Work out the finished part from the listing and answer in its coordinate system (mm). Face numbers are marked on the shaded views. A direction names the side the tool comes from. Round coordinates to 2 decimals unless told otherwise and drop trailing zeros. Loops run counter-clockwise (first coordinate to the right, second up) from the corner with the lowest first, then second, coordinate; pieces in that order, holes last. Notation, with made-up numbers: (23.25, -23.5) -> (38.25, -23.5) arc R24 cw to (38.25, 11.5) -> close; hole circle Ø8 at (59.5, -20.75). An arc over 180 degrees is marked (long way). Use one line per item in the form item = value.
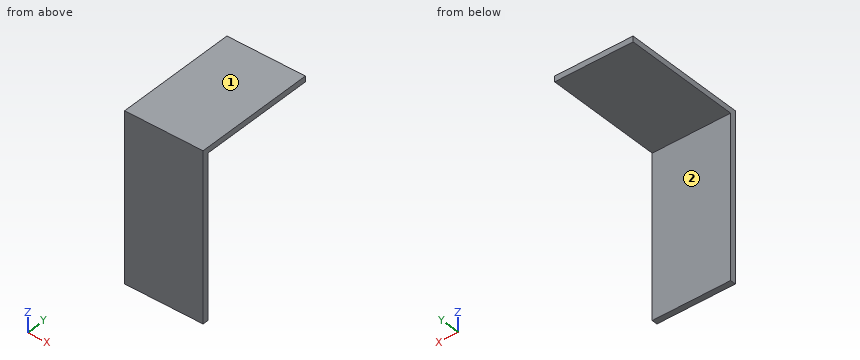
```python
from build123d import *

# Parameters (mm, degrees)
F0_W     = 250
F0_H     = 517
F1_DEPTH = 18
F2_W     = 250
F2_H     = 18
F3_DEPTH = 390


with BuildPart() as f1:
    # F0 (on Front) → F1 (new body)
    with BuildSketch(Plane.XZ):
        with Locations((125, 258.5)):
            Rectangle(F0_W, F0_H)
    extrude(amount=F1_DEPTH)

    # F2 (on face) → F3 (join)
    with BuildSketch(Plane.XZ.offset(18)):
        with Locations((125, 526)):
            Rectangle(F2_W, F2_H)
    extrude(amount=-F3_DEPTH)


solid = f1.part
```
(1) Find section C-C, the plane y = 57. Write down the section's boundary in (x, z), then the cut area to 3 significant figures.
Completed:
outline = (0, 517) -> (250, 517) -> (250, 535) -> (0, 535) -> close
area = 4,500 mm2
(2) Find section A-A, the plane x = 141. Write down the section's boundary in (y, z).
Completed:
outline = (-18, 0) -> (0, 0) -> (0, 517) -> (372, 517) -> (372, 535) -> (-18, 535) -> close
(3) Given P1, Ø8, axis at x = 180, y = 173.5, coming from the -Z side; P2, Ø3, axis at x = 31, z = 389.5, coming from the +Y side, each flat-ended and moving along its own axis, determine where each tip first touches the part or whether it passes through.
Completed:
P1 = 517
P2 = 0
(4) Consider L1, parallel to Z at x = 207.5, y = 13.5; L2, parallel to Y at x = 61.5, z = 245. Determine where each line is inside the solid, lowest interval first.
Completed:
L1 = 517 to 535
L2 = -18 to 0
(5) For the marked faces 1 and 2, determine the directions among +Z, -Z, +X, -X, +Y, -Y from which every point of the face is accessible in a straight line to the end or side of a thin tool.
Completed:
face_1 = +Z, +X, -X, +Y, -Y
face_2 = -Z, +X, -X, +Y
(6) Find section B-B, the plane z = 39. Write down the section's boundary in (x, y).
Completed:
outline = (0, -18) -> (250, -18) -> (250, 0) -> (0, 0) -> close
